For this review, take the finished solid that the model builds, in its own axes (mm). A direction names the side the tool comes from. Round coordinates to 2 decimals unless told otherwise and drop trailing zeros. Order: outer loops, then holes, each group sorted by start corner. A loop starts at its lowest first (then second) coordinate and runs counter-clockwise, first axis right, second up. Notation, with made-up numbers: (81, 22.25) -> (91, 22.25) arc R31 ccw to (91, 50.25) -> close; hole circle Ø9 at (19.5, 52). An arc over 180 degrees is marked (long way). Use a Markdown table: item, result. Add a question column.
1) Consider section D-D (x = 2.1). Give the number of separate pieces and of enclosed holes in the cut face, plus the area to 3 significant figures.
2) Consider section C-C (z = -127). State the section outline as (x, y) points, plus the area to 3 significant figures.
3) Wall thickness on line 1 along Y through (x, z) = (0.9, -63.5); line 2 along Y through (x, z) = (0.9, -127); line 3 along Z through (x, y) = (2.1, 50): over which ranges is each line inside the solid? List them lowest first. Write a range as [from, to].
4) Machinability: for faces 4 (the face through (1.252, 22.515, -136.579)), 5 (the face through (1.3, 74.6, -52.6)), which of the approach directions +Z, -Z, +X, -X, +Y, -Y give a long, thin tool a straight path to every point of the face, cutting with its end or side? Answer none if there is none.
5) Consider section A-A (z = -63.5). State the section outline as (x, y) points, plus the area to 3 significant figures.
6) Consider section B-B (y = -6). State the section outline as (x, z) points, plus the area to 3 significant figures.
7) Draft analysis for pull direction Y (two halves, no side actions). For faces 1 (the face through (1.252, 58.57, -157.986)), 2 (the face through (1.25, 66.91, -170.33)), 3 (the face through (1.252, -19.045, 0.419)), state which applies: pulls with the +Y half, pulls with the -Y half, needs draft (parallel to the pull), parting line crosses it, or undercut.
8) Clearance check with flat-ended pins moving along their axes: P1, Ø1.3, axis at x = 2, z = -91.5, coming from the -Y side; P2, Ø1, axis at x = 1, z = -29.5, coming from the -Y side; P3, Ø4, axis at y = 66.31, z = -21.63, coming from the -X side; P4, Ø1.5, axis at x = 1.5, z = -142.5, coming from the +Y side. State where each tip first meets the part, or that it passes through.
```python
from build123d import *

# Parameters (mm, degrees)
BOSS_EXTRUDE1_DEPTH     = 2.54
F_1_4_CLEARANCE_HOLE1_D = 6.7564
F_8_CLEARANCE_HOLE2_D   = 4.4958


with BuildPart() as part:
    # Sketch1 → Boss-Extrude1 (new body)
    with BuildSketch(Plane(origin=(0, 0, 0), x_dir=(0, 0, -1), z_dir=(1, 0, 0))):
        with BuildLine():
            Line((50.546, 31.496), (114.554, 31.496))
            ThreePointArc((114.554, 31.496), (136.82503518, 22.27103518), (146.05, 0))
            ThreePointArc((146.05, 0), (165.1, -19.05), (184.15, 0))
            Line((184.15, 0), (184.15, 40.072825067))
            ThreePointArc((184.15, 40.072825067), (182.836868766, 48.134013135), (179.03324779, 55.36170531))
            Line((179.03324779, 55.36170531), (161.374573217, 78.788880244))
            ThreePointArc((161.374573217, 78.788880244), (152.423192921, 86.232108989), (141.091325427, 88.9))
            Line((141.091325427, 88.9), (36.810551917, 88.9))
            ThreePointArc((36.810551917, 88.9), (27.119806989, 86.978702323), (18.895109756, 81.505469508))
            Line((18.895109756, 81.505469508), (-11.56544216, 51.197220351))
            ThreePointArc((-11.56544216, 51.197220351), (-17.104341079, 42.941309016), (-19.05, 33.191750843))
            Line((-19.05, 33.191750843), (-19.05, 0))
            ThreePointArc((-19.05, 0), (0, -19.05), (19.05, 0))
            ThreePointArc((19.05, 0), (28.27496482, 22.27103518), (50.546, 31.496))
        make_face()
    extrude(amount=BOSS_EXTRUDE1_DEPTH)

    # 1/4 Clearance Hole1 (through all)
    with Locations(Plane(origin=(2.54, 0, 0), x_dir=(0, 0, -1), z_dir=(1, 0, 0))):
        with Locations((50.8, 50.546), (127, 50.546), (165.1, 0), (0, 0)):
            Hole(F_1_4_CLEARANCE_HOLE1_D / 2)

    # #8 Clearance Hole2 (through all)
    with Locations(Plane(origin=(2.54, 0, 0), x_dir=(0, 0, -1), z_dir=(1, 0, 0))):
        with Locations((76.2, 75.946), (88.9, 75.946), (101.6, 75.946), (21.625289632, 66.306331256), (12.622554878, 57.348610175), (3.619820124, 48.390889095), (152.417846487, 69.57247655), (160.062286608, 59.430852655), (167.70672673, 49.28922876), (63.5, 75.946), (50.8, 75.946), (114.3, 75.946), (127, 75.946)):
            Hole(F_8_CLEARANCE_HOLE2_D / 2)


solid = part.part
```
Results list:
| question | item | result |
|---|---|---|
| 1 | separate pieces | 1 |
| 1 | enclosed holes | 17 |
| 1 | area | 13,600 mm2 |
| 2 | outline | (0, 28.93) -> (2.54, 28.93) -> (2.54, 47.17) -> (0, 47.17) -> close; (0, 53.92) -> (2.54, 53.92) -> (2.54, 73.7) -> (0, 73.7) -> close; (0, 78.19) -> (2.54, 78.19) -> (2.54, 88.9) -> (0, 88.9) -> close |
| 2 | area | 124 mm2 |
| 3 | line 1 | [31.5, 73.7], [78.19, 88.9] |
| 3 | line 2 | [28.93, 47.17], [53.92, 73.7], [78.19, 88.9] |
| 3 | line 3 | [-182.13, -169.84], [-165.57, -130.33], [-123.67, -54.13], [-47.47, -5.19], [-2.05, 12.69] |
| 4 | face 4 | +X, -X, -Y |
| 4 | face 5 | +X, -X |
| 5 | outline | (0, 31.5) -> (2.54, 31.5) -> (2.54, 73.7) -> (0, 73.7) -> close; (0, 78.19) -> (2.54, 78.19) -> (2.54, 88.9) -> (0, 88.9) -> close |
| 5 | area | 134 mm2 |
| 6 | outline | (0, -183.18) -> (2.54, -183.18) -> (2.54, -147.02) -> (0, -147.02) -> close; (0, -18.08) -> (2.54, -18.08) -> (2.54, 18.08) -> (0, 18.08) -> close |
| 6 | area | 184 mm2 |
| 7 | face 1 | undercut |
| 7 | face 2 | pulls with the +Y half |
| 7 | face 3 | pulls with the -Y half |
| 8 | P1 | y = 31.5 |
| 8 | P2 | y = 22.97 |
| 8 | P3 | through |
| 8 | P4 | y = 88.89 |
